For this review, take the finished solid that the model builds, in its own axes (mm). A direction names the side the tool comes from. Give positions to 0.01 mm unless a question says otherwise; leave off trailing zeros. Write each loop counter-clockwise with the first axis right and the second up, starting at its lowest first coordinate (ties: lowest second). Pieces come first, ordered by that corner, then holes. Notation, with made-up numbers: M 67,1 L 115,1 A19 ccw 115,10 Z; hole C -12,-21 d10. An arc over 180 degrees is marked long. Write item = value, one per line.
```python
from build123d import *

# Parameters (mm, degrees)
F1_DEPTH = 20
F2_R     = 2
F3_T     = -3
F4_R     = 1
F5_R     = 2


with BuildPart() as f1:
    # F0 (on Top) → F1 (new body)
    with BuildSketch(Plane.XY):
        with BuildLine():
            Line((8, 10), (-8, 10))
            ThreePointArc((-8, 10), (-9.4142135624, 9.4142135624), (-10, 8))
            Line((-10, 8), (-10, -8))
            ThreePointArc((-10, -8), (-9.4142135624, -9.4142135624), (-8, -10))
            Line((-8, -10), (8, -10))
            ThreePointArc((8, -10), (9.4142135624, -9.4142135624), (10, -8))
            Line((10, -8), (10, 8))
            ThreePointArc((10, 8), (9.4142135624, 9.4142135624), (8, 10))
        make_face()
    extrude(amount=F1_DEPTH)

    # F2
    f2_edges = [f1.edges().sort_by_distance(p)[0] for p in [
        (0, -10, 0),
    ]]
    fillet(f2_edges, radius=F2_R)

    # F3
    f3_openings = [f1.faces().sort_by_distance(p)[0] for p in [
        (0, 0, 20),
    ]]
    offset(amount=F3_T, openings=f3_openings)

    # F4
    f4_edges = [f1.edges().sort_by_distance(p)[0] for p in [
        (-10, 0, 20),
        (7, 0, 20),
        (0, 7, 20),
        (-7, 0, 20),
        (0, -7, 20),
        (0, 10, 20),
        (9.414214, 9.414214, 20),
        (-9.414214, 9.414214, 20),
        (10, 0, 20),
        (-9.414214, -9.414214, 20),
        (0, -10, 20),
        (9.414214, -9.414214, 20),
    ]]
    fillet(f4_edges, radius=F4_R)

    # F5
    f5_edges = [f1.edges().sort_by_distance(p)[0] for p in [
        (7, 0, 3),
        (0, -7, 3),
        (0, 7, 3),
        (-7, 0, 3),
    ]]
    fillet(f5_edges, radius=F5_R)


solid = f1.part
```
1. We need section A-A, the plane z = 9.25. Write out the cut boundary in (x, y), then the cut area to 3 significant figures.
Responses:
outline = M -10,-8 A2 ccw -8,-10 L 8,-10 A2 ccw 10,-8 L 10,8 A2 ccw 8,10 L -8,10 A2 ccw -10,8 Z; hole M -7,-7 L 7,-7 L 7,7 L -7,7 Z
area = 201 mm2
2. The part is to be moulded in two halves that separate along X. For faces 1 (the face through (-6.43, -0.1, 3.6)), 2 (the face through (0.11, -9.43, 0.6)), 3 (the face through (10, 0, 10)), say which applies: +X half, -X half, draft (parallel to the pull), parting line (faces both ways), or undercut.
Responses:
face_1 = undercut
face_2 = draft
face_3 = +X half
3. Machinability: for faces 4 (the face through (9.43, 9.4, 10.38)), 5 (the face through (-0.112, 7.301, 19.715)), which of the approach directions +Z, -Z, +X, -X, +Y, -Y give a long, thin tool a straight path to every point of the face, cutting with its end or side? Answer none if there is none.
Responses:
face_4 = +Z, -Z, +X, +Y
face_5 = +Z
4. For line 1 along Y through (x, z) = (-6.5, 18); line 2 along Z through (x, y) = (2.25, 3.5), list the stretches that pass through material, from the lowest coordinate up. Write a range as from..to.
Responses:
line_1 = -10..-7, 7..10
line_2 = 0..3
5. We need section B-B, the plane y = -2. Write out the cut boundary in (x, z), then the cut area to 3 significant figures.
Responses:
outline = M -10,2 A2 ccw -8,0 L 8,0 A2 ccw 10,2 L 10,19 A1 ccw 9,20 L 8,20 A1 ccw 7,19 L 7,5 A2 cw 5,3 L -5,3 A2 cw -7,5 L -7,19 A1 ccw -8,20 L -9,20 A1 ccw -10,19 Z
area = 161 mm2
